```python
from build123d import *

# Parameters (mm, degrees)
FILLET1_R           = 0.8
FILLET2_R           = 0.5
SKETCH2_R           = 3
BOSS_EXTRUDE1_DEPTH = 0.5


with BuildPart() as part:
    # Sketch1 → Revolve1 (revolve)
    with BuildSketch(Plane.XY, mode=Mode.PRIVATE) as revolve1_sk:
        with BuildLine():
            Line((-1.5, 1), (-2.2, 1))
            ThreePointArc((-2.2, 1), (-1.65, 1.227674865), (-1.1, 1))
            Line((-1.1, 1), (-1.1, -0.762073649))
            Line((-1.1, -0.762073649), (0, -0.924951874))
            Line((0, -0.924951874), (0, -1.1))
            Line((0, -1.1), (-1.5, -1.1))
            Line((-1.5, -1.1), (-1.5, 1))
        make_face()
    revolve(revolve1_sk.sketch.rotate(Axis((0, -1.1, 0), (0, 1, 0)), 180), axis=Axis((0, -1.1, 0), (0, 1, 0)))

    # Fillet1
    fillet1_edges = [part.edges().sort_by_distance(p)[0] for p in [
        (-1.1, -0.762073649, 0),
    ]]
    fillet(fillet1_edges, radius=FILLET1_R)

    # Fillet2
    fillet2_edges = [part.edges().sort_by_distance(p)[0] for p in [
        (-1.1, 1, 0),
    ]]
    fillet(fillet2_edges, radius=FILLET2_R)

    # Sketch2 → Boss-Extrude1 (add)
    with BuildSketch(Plane.XZ.offset(1.1)):
        Circle(SKETCH2_R)
    extrude(amount=BOSS_EXTRUDE1_DEPTH)


solid = part.part
```
Here's how the part is built. I have some questions about the finished solid (model axes, mm). A direction names the side the tool comes from. Give positions to 0.01 mm unless a question says otherwise; leave off trailing zeros. Loops run counter-clockwise (first coordinate to the right, second up) from the corner with the lowest first, then second, coordinate; pieces in that order, holes last. Notation, with made-up numbers: M 76,34 L 113,34 A20 ccw 113,53 Z; hole C 9,34 d9. An arc over 180 degrees is marked long. Put each result on its own line as item: value. Start each with the question number.
(1) I want a section at B-B on z = -2.55. Please give me the cut outline in (x, y), then the cut area to 3 significant figures.
(2) I want a section at A-A on y = 0.6. Please give me the cut outline in (x, z), then the cut area to 3 significant figures.
(3) For faces 1 (the cylindrical face through (-3, -1.3, 0.1)), 2 (the flat face through (-0.9, 1, 1.4)), which set-ups out of +Z, -Z, +X, -X, +Y, -Y let a thin tool reach every point of the face, with its end or its side?
(4) If we mould it in two halves opening along Z, with no side actions, what happens to faces 3 (the cylindrical face through (1.43, -0.04, -0.45)), 4 (the flat face through (1.3, -1.1, -1.3)), 5 (the cylindrical face through (0.508, 0.32, 0.976))? For each: +Z half, -Z half, draft (parallel to the pull), parting line (faces both ways), or undercut.
(5) I need wall thicknesses on line 1 along Z through (x, y) = (0, 0.35); line 2 along Y through (x, z) = (-1.7, 0.6); line 3 along Y through (x, z) = (-0.15, 0.4). Which ranges of each line are inside material? Lowest first, please. Write a range as [from, to].
(6) I want a section at C-C on x = -2.45. Please give me the cut outline in (y, z), then the cut area to 3 significant figures.
Answer block:
1. outline: M -1.58,-1.6 L 1.58,-1.6 L 1.58,-1.1 L -1.58,-1.1 Z
1. area: 1.58 mm^2
2. outline: C 0,0 d3; hole C 0,0 d2.2
2. area: 3.27 mm^2
3. face 1: +Y, -Y
3. face 2: none
4. face 3: parting line
4. face 4: draft
4. face 5: undercut
5. line 1: [-1.5, -1.1], [1.1, 1.5]
5. line 2: [-1.6, -1.1], [1, 1.21]
5. line 3: [-1.6, -0.86]
6. outline: M -1.6,-1.73 L -1.1,-1.73 L -1.1,1.73 L -1.6,1.73 Z
6. area: 1.73 mm^2
